The model under review builds one solid part; all positions refer to its coordinate system, in mm. A direction names the side the tool comes from. Give positions to 0.01 mm unless a question says otherwise; leave off trailing zeros. Loops run counter-clockwise (first coordinate to the right, second up) from the corner with the lowest first, then second, coordinate; pieces in that order, holes last. Notation, with made-up numbers: M 10.5,60 L 44.5,60 A20 ccw 44.5,82 Z; hole C 84.25,36 d4. An arc over 180 degrees is marked long. Return JSON: item names as keys, results as strings.
```python
from build123d import *

# Parameters (mm, degrees)
CIRPATTERN1_COUNT  = 2
CIRPATTERN1_ANGLE  = 90
SKETCH5_R          = 2.69875
CUT_EXTRUDE3_DEPTH = 29.211156942
SKETCH6_R          = 2.69875
CUT_EXTRUDE4_DEPTH = 29.211156942
REVOLVE2_ANGLE     = 90
FILLET1_R          = 0.254


with BuildPart() as part:
    # Sketch1 → Revolve1 (revolve)
    with BuildSketch(Plane.XY):
        with BuildLine():
            Line((-15.24, 7.112), (-9.652, 7.112))
            Line((-9.652, 7.112), (-8.128451706, 6.0452))
            Line((-8.128451706, 6.0452), (0, 6.0452))
            Line((0, 6.0452), (0, 2.69875))
            Line((0, 2.69875), (-9.652, 2.69875))
            Line((-9.652, 2.69875), (-9.652, 3.175))
            Line((-9.652, 3.175), (-18.923, 3.175))
            Line((-18.923, 3.175), (-19.304, 3.556))
            Line((-19.304, 3.556), (-19.304, 5.6388))
            ThreePointArc((-19.304, 5.6388), (-19.080815367, 6.177615367), (-18.542, 6.4008))
            Line((-18.542, 6.4008), (-17.399, 6.4008))
            Line((-17.399, 6.4008), (-17.399, 4.1275))
            Line((-17.399, 4.1275), (-15.24, 4.1275))
            Line((-15.24, 4.1275), (-15.24, 7.112))
        make_face()
    revolve1 = revolve(axis=Axis((0, 0, 0), (-1, 0, 0)))

    # CirPattern1: Revolve1 ×2 about axis
    cirpattern1_axis = Axis((0, 0, -6.0452), (0, 0, -1))
    for i in range(1, CIRPATTERN1_COUNT):
        add(revolve1.rotate(cirpattern1_axis, i * CIRPATTERN1_ANGLE / (CIRPATTERN1_COUNT - 1)))

    # Sketch5 → Cut-Extrude3 (cut, through all)
    with BuildSketch(Plane.XZ):
        Circle(SKETCH5_R)
    extrude(amount=-CUT_EXTRUDE3_DEPTH, mode=Mode.SUBTRACT)

    # Sketch6 → Cut-Extrude4 (cut, through all)
    with BuildSketch(Plane(origin=(0, 0, 0), x_dir=(0, 0, -1), z_dir=(1, 0, 0))):
        with Locations(Location((0, 0, 0), (0, 0, 90))):
            Circle(SKETCH6_R)
    extrude(amount=-CUT_EXTRUDE4_DEPTH, mode=Mode.SUBTRACT)

    # Sketch7 → Revolve2 (revolve)
    with BuildSketch(Plane(origin=(0, 0, 0), x_dir=(0, 0, -1), z_dir=(1, 0, 0))):
        with BuildLine():
            Line((-2.69875, 0), (-6.0452, 0))
            ThreePointArc((-6.0452, 0), (0, -6.0452), (6.0452, 0))
            Line((6.0452, 0), (2.69875, 0))
            ThreePointArc((2.69875, 0), (0, -2.69875), (-2.69875, 0))
        make_face()
    revolve(axis=Axis((0, 0, -2.69875), (0, 0, 1)), revolution_arc=REVOLVE2_ANGLE)

    # Fillet1
    fillet1_edges = [part.edges().sort_by_distance(p)[0] for p in [
        (-3.905494855, 3.905494855, -4.614277081),
    ]]
    fillet(fillet1_edges, radius=FILLET1_R)


solid = part.part
```
1) Tool access review of faces 1 (the face through (0, 19.304, 4)), 2 (the face through (-4.894, -2.696, -0.119)), 3 (the face through (1.5, 14.4, 2.8)), 4 (the face through (-15.24, -3.1, 3.1)): name each direction out of +Z, -Z, +X, -X, +Y, -Y from which nothing blocks a thin tool from reaching the whole face with its end or side.
From the geometry:
{"face 1": "+Z, -Z, +X, -X, +Y", "face 2": "-X", "face 3": "+Y", "face 4": "none"}
2) Wall thickness on L1, parallel to Y at x = -4, z = 0; L2, parallel to Y at x = -11.75, z = 0 (3 decimals); L3, parallel to X at y = 2.75, z = -2.25: over which ranges is each line inside the solid? List them lowest first. Write a range as from..to.
From the geometry:
{"L1": "-6.05..-2.7, 2.7..19.3", "L2": "-7.112..-3.175, 3.175..7.112", "L3": "-19.3..-1.49, 1.49..5.61"}
3) Consider section B-B on x = -11.25. Write out the cut boundary in (y, z) (3 decimals), then the cut area to 3 significant figures.
From the geometry:
{"outline": "C 0,0 d14.224; hole C 0,0 d6.35", "area": "127 mm²"}
4) Consider section A-A on y = 5. Count the separate pieces of the cut face and the enclosed holes in it, then the cut area to 3 significant figures.
From the geometry:
{"separate pieces": "2", "enclosed holes": "1", "area": "193 mm²"}
5) Insertion check: pin 1 (4 mm diameter, centred on y = 0, z = 0, fed in from +X); pin 2 (5 mm diameter, centred on y = 0.5, z = 0, fed in from -X); pin 3 (3 mm diameter, centred on x = -10.5, y = 12.5, fed in from +Z); pin 4 (2 mm diameter, centred on x = -7, y = 10.5, fed in from -Z). Each pin has a flat end and moves straight along its axis. Give the tip position at first contact, or say it passes through.
From the geometry:
{"pin 1": "x = 6.05", "pin 2": "x = -9.65", "pin 3": "through", "pin 4": "z = -3.82"}
6) The part is to be moulded in two halves that separate along X. For faces 5 (the face through (-16.304, 3.937, -1.24)), 6 (the face through (-12.407, -1.542, 6.943)), 7 (the face through (3.937, 16.304, -1.24)), say which applies: released by +X, released by -X, zero draft, split by the parting line, or undercut.
From the geometry:
{"face 5": "undercut", "face 6": "zero draft", "face 7": "split by the parting line"}
